CAD build for the part. Positions are in the model's coordinates, mm. Face numbers are marked on the shaded views. Round coordinates to 2 decimals unless told otherwise and drop trailing zeros. Write each loop counter-clockwise with the first axis right and the second up, starting at its lowest first coordinate (ties: lowest second). Pieces come first, ordered by that corner, then holes. Notation, with made-up numbers: (75, 38.5) - (114, 38.5) arc R15 cw to (114, 67.5) - close; hole circle Ø2 at (53.5, -32). An arc over 180 degrees is marked (long way). Use one line per item in the form item = value. Start each with the question number.
Item 1: Band-saw the part on C-C, the plane z = 22. List the corners of the cut face in (x, y).
Item 2: Band-saw the part on D-D, the plane z = 33. List the corners of the cut face in (x, y), and give its area (3 significant figures).
Item 3: Band-saw the part on B-B, the plane x = 175.5. List the corners of the cut face in (y, z).
Item 4: Band-saw the part on A-A, the plane y = -27.5. List the corners of the cut face in (x, z).
Item 5: Pull direction Z, two halves, no side cores. Call the marked faces 1, 2, 3 and 4: +Z half, -Z half, draft (parallel to the pull), parting line (faces both ways), or undercut.
Item 6: Pin check, flat tips, straight feed: pin 1 (12 mm diameter, centred on x = 172.5, z = 29.5, fed in from +Y); pin 2 (10 mm diameter, centred on y = -13.5, z = 24.5, fed in from -X). Stop position of each tip, or through.
Item 7: Drill centre lines: L1, parallel to Z at x = 111.5, y = -26; L2, parallel to Z at x = 150.5, y = -21; L3, parallel to Y at x = 104, z = 29. Where is each one in solid material? Low to high.
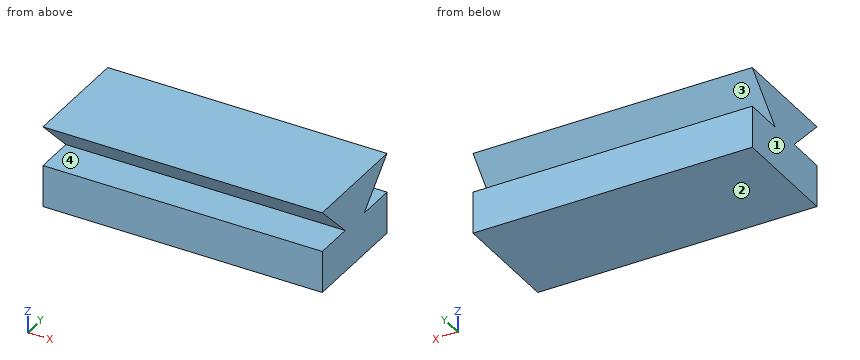
from build123d import *

# Parameters (mm, degrees)
F1_DEPTH = 200


with BuildPart() as f1:
    # F0 (on Right) → F1 (new body)
    with BuildSketch(Plane.YZ):
        Polygon((39.280485, 38.99768), (-40.719515, 38.99768), (-12.435243, 10.713409), (10.996214, 10.713409), align=None)
        Polygon((10.996214, 10.713409), (-12.435243, 10.713409), (-40.719515, 10.713409), (-40.719515, -19.286591), (39.280485, -19.286591), (39.280485, 10.713409), align=None)
    extrude(amount=F1_DEPTH)


solid = f1.part
Determined:
q1.outline = (0, -23.72) - (200, -23.72) - (200, 22.28) - (0, 22.28) - close
q2.outline = (0, -34.72) - (200, -34.72) - (200, 33.28) - (0, 33.28) - close
q2.area = 13,600 mm²
q3.outline = (-40.72, -19.29) - (39.28, -19.29) - (39.28, 10.71) - (11, 10.71) - (39.28, 39) - (-40.72, 39) - (-12.44, 10.71) - (-40.72, 10.71) - close
q4.outline = (0, -19.29) - (200, -19.29) - (200, 10.71) - (0, 10.71) - close; (0, 25.78) - (200, 25.78) - (200, 39) - (0, 39) - close
q5.face_1 = draft
q5.face_2 = -Z half
q5.face_3 = undercut
q5.face_4 = undercut
q6.pin_1 = 35.78
q6.pin_2 = 0
q7.L1 = -19.29 to 10.71, 24.28 to 39
q7.L2 = -19.29 to 10.71, 19.28 to 39
q7.L3 = -30.72 to 29.28
